Source: CAD feature listing. Evaluate the final solid. Frame: model axes, mm. Face numbers are marked on the shaded views. Round coordinates to 2 decimals unless told otherwise and drop trailing zeros. Write each loop counter-clockwise with the first axis right and the second up, starting at its lowest first coordinate (ties: lowest second). Pieces come first, ordered by that corner, then holes. Notation, with made-up numbers: M 63.5,-8 L 101.5,-8 A11 cw 101.5,1 Z; hole C 29.5,62 d4. An arc over 180 degrees is marked long. Use a Markdown table: item, result.
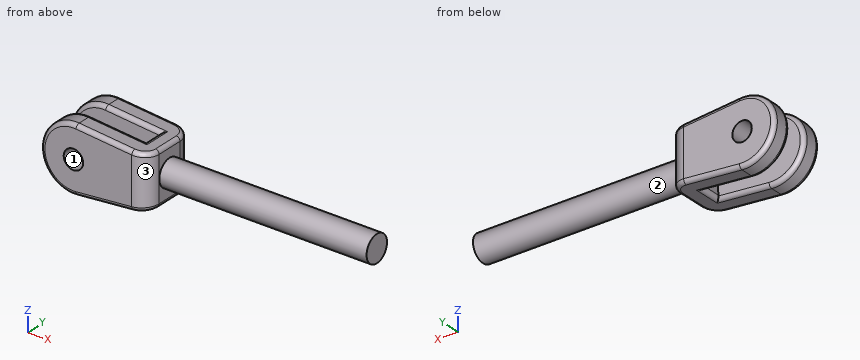
```python
from build123d import *

# Parameters (mm, degrees)
SKETCH4_R               = 2.619375
BOSS_EXTRUDE2_DEPTH     = 40.64
BOSS_EXTRUDE4_DEPTH     = 5.715
CUT_EXTRUDE2_DEPTH      = 43.16105899
CUT_EXTRUDE2_DEPTH_BACK = 43.16105899
SKETCH16_W              = 25.774361669
SKETCH16_H              = 3.81
CUT_EXTRUDE3_DEPTH      = 43.691650237
CUT_EXTRUDE3_DEPTH_BACK = 43.691650237
SKETCH17_R              = 1.905
FILLET1_R               = 3.048
FILLET2_R               = 0.762
SCALE1_SCALE            = 6


with BuildPart() as part:
    # Sketch4 → Boss-Extrude2 (new body)
    with BuildSketch(Plane(origin=(0, 0, 0), x_dir=(0, 0, -1), z_dir=(1, 0, 0))):
        Circle(SKETCH4_R)
    extrude(amount=BOSS_EXTRUDE2_DEPTH)

    # Sketch13 → Boss-Extrude4 (add, symmetric)
    with BuildSketch(Plane(origin=(0, 0, 0), x_dir=(1, 0, 0), z_dir=(0, 1, 0))):
        with BuildLine():
            Line((0, 5.08), (0, -5.08))
            Line((0, -5.08), (-13.91443545, -6.324743387))
            ThreePointArc((-13.91443545, -6.324743387), (-20.830227899, 0), (-13.91443545, 6.324743387))
            Line((-13.91443545, 6.324743387), (0, 5.08))
        make_face()
    extrude(amount=BOSS_EXTRUDE4_DEPTH, both=True)

    # Sketch16 → Cut-Extrude2 (cut, two sides: drawn at the far end of the back side and taken through both)
    with BuildSketch(Plane(origin=(0.450833644, 0, 5.039669783), x_dir=(0.996022580554145, 0, -0.08910117297915686), z_dir=(0.08910117297915686, 0, 0.996022580554145)).offset(-CUT_EXTRUDE2_DEPTH_BACK)):
        with Locations((-16.514814794, 0)):
            Rectangle(SKETCH16_W, SKETCH16_H)
    extrude(amount=CUT_EXTRUDE2_DEPTH + CUT_EXTRUDE2_DEPTH_BACK, mode=Mode.SUBTRACT)

    # Sketch17 → Cut-Extrude3 (cut, two sides: drawn at the far end of the back side and taken through both)
    with BuildSketch(Plane.XZ.offset(5.715).offset(-CUT_EXTRUDE3_DEPTH_BACK)):
        with Locations(Location((-14.480227899, 0, 0), (0, 0, 270))):
            Circle(SKETCH17_R)
    extrude(amount=CUT_EXTRUDE3_DEPTH + CUT_EXTRUDE3_DEPTH_BACK, mode=Mode.SUBTRACT)

    # Fillet1
    fillet1_edges = [part.edges().sort_by_distance(p)[0] for p in [
        (0, -5.715, 0),
        (0, 5.715, 0),
    ]]
    fillet(fillet1_edges, radius=FILLET1_R)

    # Fillet2
    fillet2_edges = [part.edges().sort_by_distance(p)[0] for p in [
        (-8.538403572, -1.905, 5.843819805),
        (-3.162371693, 0, 5.362896224),
        (-8.538403572, 1.905, 5.843819805),
        (-9.02202226, 1.905, -5.887082873),
        (-20.830227899, 1.905, 0),
        (-4.12960907, 0, -5.44942236),
        (-20.830227899, -1.905, 0),
        (-9.02202226, -1.905, -5.887082873),
        (0, 0, -5.08),
        (0, 0, 5.08),
        (-8.481217725, 5.715, -5.838704132),
        (-8.481217725, -5.715, -5.838704132),
        (-0.894886956, 4.824407754, -5.160053885),
        (-0.894886956, -4.824407754, -5.160053885),
        (-0.894886956, 4.824407754, 5.160053885),
        (-0.894886956, -4.824407754, 5.160053885),
        (-20.830227899, -5.715, 0),
        (-8.481217725, -5.715, 5.838704132),
        (-20.830227899, 5.715, 0),
        (-8.481217725, 5.715, 5.838704132),
    ]]
    fillet(fillet2_edges, radius=FILLET2_R)


with BuildPart() as part_1:
    # Scale1: scaled about (0.503603853, 0, -0.013653442)
    add(part.part.scale(SCALE1_SCALE).moved(Location((-2.518019265, 0, 0.06826721))))


solid = part_1.part
```
Q1. First-contact query: pin 1 Ø10 at (y, z) = (-22.5, 21) entering from +X; pin 2 Ø2 at (x, z) = (191, 15.5) entering from -Y; pin 3 Ø2 at (y, z) = (21.5, 30.5) entering from +X; pin 4 Ø20.5 at (x, z) = (-89.4, 0.07) entering from +Y. Flat tips, straight axial feed; report the tip coordinate or a pass-through.
Results are:
| item | result |
|---|---|
| pin 1 | x = -2.58 |
| pin 2 | y = -6.22 |
| pin 3 | x = -4.56 |
| pin 4 | through |
Q2. Line query: L1, parallel to Y at x = -83, z = -32; L2, parallel to Z at x = -82.5, y = 12.5; L3, parallel to Y at x = -110.5, z = -27. Output: solid intervals per line, ascending.
Results are:
| item | result |
|---|---|
| L1 | -34.29 to -11.43, 11.43 to 34.29 |
| L2 | -35.93 to -9.04, 9.18 to 36.06 |
| L3 | -34.22 to -11.5, 11.5 to 34.22 |
Q3. Section A-A on y = 0. Return loops of the section in (x, z), plus the area to 3 significant figures.
Results are:
| item | result |
|---|---|
| outline | M -26.81,-27.18 A4.57 ccw -21.85,-32.14 L -6.68,-30.78 A4.57 ccw -2.52,-26.23 L -2.52,-15.65 L 241.32,-15.65 L 241.32,15.78 L -2.52,15.78 L -2.52,26.37 A4.57 ccw -6.68,30.92 L -16.94,31.84 A4.57 ccw -21.9,27.69 Z |
| area | 9,020 mm^2 |
Q4. Mould query, pull axis Z, two halves, no side actions, for the marked faces 1, 2 and 3. Classes: +Z half, -Z half, draft (parallel to the pull), parting line (faces both ways), or undercut.
Results are:
| item | result |
|---|---|
| face 1 | undercut |
| face 2 | parting line |
| face 3 | draft |
Q5. Section B-B on x = 2. Return loops of the section in (y, z), plus the area to 3 significant figures.
Results are:
| item | result |
|---|---|
| outline | C 0,0.07 d31.43 |
| area | 776 mm^2 |
